```python
from build123d import *

# Parameters (mm, degrees)
BOSS_EXTRUDE1_DEPTH = 6
SHELL1_START        = 2
SHELL1_DEPTH        = 2
FILLET1_R           = 1.5


# Read off the part's stored shape, not the designer's step: Shell1
with BuildPart() as part:
    # Sketch1 → Boss-Extrude1 (new body)
    with BuildSketch(Plane(origin=(0, 0, 0), x_dir=(1, 0, 0), z_dir=(0, 1, 0))):
        with BuildLine():
            Line((0, 0), (17.207293091, 24.574561329))
            Line((17.207293091, 24.574561329), (23.445639192, 12.590809966))
            Line((23.445639192, 12.590809966), (4.341304412, 2.645722757))
            ThreePointArc((4.341304412, 2.645722757), (4.195782463, 2.184186102), (4.657319118, 2.038664153))
            Line((4.657319118, 2.038664153), (23.761653899, 11.983751363))
            Line((23.761653899, 11.983751363), (30, 0))
            Line((30, 0), (0, 0))
        make_face()
    extrude(amount=BOSS_EXTRUDE1_DEPTH)

    # Shell1 outline → Shell1 (cut)
    with BuildSketch(Plane(origin=(0, 0, 0), x_dir=(1, 0, 0), z_dir=(0, 1, 0)).offset(SHELL1_START)):
        Polygon((4.321177127, 2.68438691), (4.341304412, 2.645722757), (23.445639192, 12.590809966), (18.248427192, 22.574561329), align=None)
        Polygon((23.761653899, 11.983751363), (4.657319118, 2.038664153), (4.677446402, 2), (28.958865899, 2), align=None)
    extrude(amount=SHELL1_DEPTH, mode=Mode.SUBTRACT)

    # Fillet1
    fillet1_edges = [part.edges().sort_by_distance(p)[0] for p in [
        (0, 3, 0),
    ]]
    fillet(fillet1_edges, radius=FILLET1_R)


solid = part.part
```
For this review, take the finished solid that the model builds, in its own axes (mm). A direction names the side the tool comes from. Round coordinates to 2 decimals unless told otherwise and drop trailing zeros. Order: outer loops, then holes, each group sorted by start corner. A loop starts at its lowest first (then second) coordinate and runs counter-clockwise, first axis right, second up.
Q1. Mouldability with a two-part tool opening along X and no side actions: class faces 1 (the flat face through (19, 2, -5)), 2 (the flat face through (14.03, 4.99, -7.69)), 3 (the flat face through (11.382, 2.986, -12.769)) as pulls with the +X half, pulls with the -X half, needs draft (parallel to the pull), parting line crosses it, or undercut.
Findings below:
face 1: needs draft
face 2: undercut
face 3: pulls with the +X half
Q2. We need section B-B, the plane y = 2.6. Give the boundary of the cut face in (x, z).
Findings below:
outline: (1.65, -2.36) - (17.21, -24.57) - (18.25, -22.57) - (4.32, -2.68) - (4.34, -2.65) arc R0.34 cw to (4.66, -2.04) - (4.68, -2) - (28.96, -2) - (30, 0) - (2.88, 0) arc R1.5 ccw to start
Q3. We need section C-C, the plane z = -3.75. Give the boundary of the cut face in (x, y).
Findings below:
outline: (2.63, 0) - (6.46, 0) - (6.46, 2) - (5.07, 2) - (5.07, 4) - (6.46, 4) - (6.46, 6) - (2.63, 6) - close; (7.94, 0) - (28.05, 0) - (28.05, 2) - (7.94, 2) - close; (7.94, 4) - (28.05, 4) - (28.05, 6) - (7.94, 6) - close
Q4. We need section D-D, the plane x = 19. Give the boundary of the cut face in (y, z) (3 decimals), plus the area to 3 significant figures.
Findings below:
outline: (0, -21.131) - (2, -21.131) - (2, -10.277) - (0, -10.277) - close; (0, -9.505) - (2, -9.505) - (2, -2) - (4, -2) - (4, -9.505) - (6, -9.505) - (6, 0) - (0, 0) - close; (4, -21.131) - (6, -21.131) - (6, -10.277) - (4, -10.277) - close
area: 85.4 mm2
Q5. Machinability: for faces 4 (the flat face through (17, 3, -2)), 5 (the flat face through (14.03, 0.99, -7.69)), 6 (the flat face through (9.32, 2.96, -13.31)), which of the approach directions +Z, -Z, +X, -X, +Y, -Y give a long, thin tool a straight path to every point of the face, cutting with its end or side? Answer none if there is none.
Findings below:
face 4: +X
face 5: +Y, -Y
face 6: -Z, -X, +Y, -Y
Q6. We need section A-A, the plane x = 14.75. Give the boundary of the cut face in (y, z).
Findings below:
outline: (0, -21.07) - (6, -21.07) - (6, -8.06) - (4, -8.06) - (4, -17.58) - (2, -17.58) - (2, -8.06) - (0, -8.06) - close; (0, -7.29) - (2, -7.29) - (2, -2) - (4, -2) - (4, -7.29) - (6, -7.29) - (6, 0) - (0, 0) - close
Q7. Wall thickness on line 1 (Y direction, x = 15.5, z = -4.25); line 2 (Z direction, x = 10, y = 3.8); line 3 (Z direction, x = 27.5, y = 2.35): over which ranges is each line inside the solid? List them lowest first.
Findings below:
line 1: y = 0 to 2, 4 to 6
line 2: z = -14.28 to -10.79, -2 to 0
line 3: z = -2 to 0
Q8. Insertion check: P1, Ø0.6, axis at x = 21.5, y = 3, coming from the -Z side; P2, Ø5.5, axis at x = 18, z = -15.5, coming from the -Y side; P3, Ø3, axis at y = 1, z = -19.5, coming from the -X side; P4, Ø2, axis at x = 12.5, y = 2.5, coming from the -Z side. Each pin has a flat end and moves straight along its axis. Give the tip position at first contact, or say it passes through.
Findings below:
P1: stops at z = -2
P2: stops at y = 0
P3: stops at x = 12.6
P4: stops at z = -19.28
